Input: dimensioned drawing with shaded views. Units: mm. Origin: part minimum x, y, z. Give positions to 0.01 mm unless a question says otherwise; leave off trailing zeros. Order: outer loops, then holes, each group sorted by start corner. A loop starts at its lowest first (then second) coordinate and runs counter-clockwise, first axis right, second up.
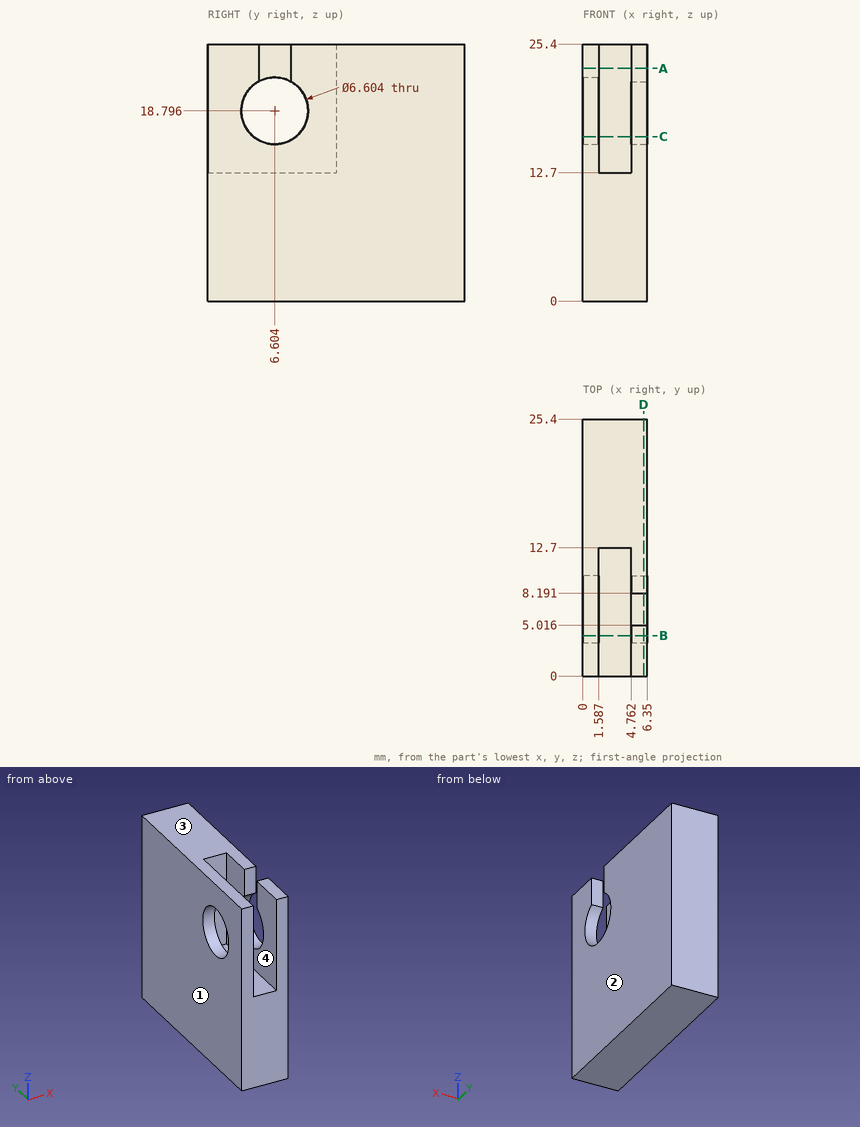
1) Section query A-A, the plane z = 23. Return the cut outline in (x, y), and give its area (3 significant figures).
Report:
outline: (0, 0) - (1.59, 0) - (1.59, 12.7) - (4.76, 12.7) - (4.76, 8.19) - (6.35, 8.19) - (6.35, 25.4) - (0, 25.4) - close; (4.76, 0) - (6.35, 0) - (6.35, 5.02) - (4.76, 5.02) - close
area: 116 mm2
2) Draft query along X for the marked faces 1, 2, 3 and 4. Return one class per face: +X half, -X half, draft (parallel to the pull), parting line (faces both ways), or undercut.
Report:
face 1: -X half
face 2: +X half
face 3: draft
face 4: undercut
3) Pin query (flat end, axial travel): pin 1 (1.6 mm diameter, centred on x = 3.5, z = 22, fed in from -Y); pin 2 (1.5 mm diameter, centred on x = 3, y = 7, fed in from +Z). Return the tip coordinate at first contact, or that it passes through.
Report:
pin 1: stops at y = 12.7
pin 2: stops at z = 12.7
4) Section query B-B, the plane y = 4. Count the separate pieces of the cut face and the enclosed holes in it, and give its area (3 significant figures).
Report:
separate pieces: 3
enclosed holes: 0
area: 108 mm2
5) Section query C-C, the plane z = 16.25. Return the cut outline in (x, y), and give its area (3 significant figures).
Report:
outline: (0, 0) - (1.59, 0) - (1.59, 4.5) - (0, 4.5) - close; (0, 8.71) - (1.59, 8.71) - (1.59, 12.7) - (4.76, 12.7) - (4.76, 8.71) - (6.35, 8.71) - (6.35, 25.4) - (0, 25.4) - close; (4.76, 0) - (6.35, 0) - (6.35, 4.5) - (4.76, 4.5) - close
area: 108 mm2
6) Section query D-D, the plane x = 6. Return the cut outline in (y, z) (1 decimal).
Report:
outline: (0, 0) - (25.4, 0) - (25.4, 25.4) - (8.2, 25.4) - (8.2, 21.7) arc R3.3 cw (long way) to (5, 21.7) - (5, 25.4) - (0, 25.4) - close
7) Material intervals for L1, parallel to X at y = 2.25, z = 12.75; L2, parallel to Y at x = 5.5, z = 24.25; L3, parallel to Z at x = 0.75, y = 6.5 (1 decimal), sorted ascending.
Report:
L1: x = 0 to 1.59, 4.76 to 6.35
L2: y = 0 to 5.02, 8.19 to 25.4
L3: z = 0 to 15.5, 22.1 to 25.4
